The listing builds one solid part. Answer for the finished solid, in the listing's coordinates (mm). Give positions to 0.01 mm unless a question says otherwise; leave off trailing zeros. Loops run counter-clockwise (first coordinate to the right, second up) from the corner with the lowest first, then second, coordinate; pieces in that order, holes last. Notation, with made-up numbers: (14.25, 20) - (54.25, 20) arc R21 ccw to (54.25, 46) - close; hole circle Ø8 at (-25.75, -2.5). An arc over 180 degrees is marked (long way). Write each question's results on one line, items separated by ' | '.
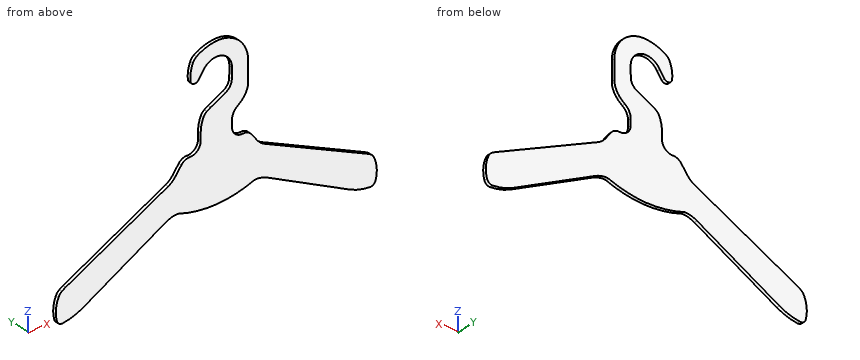
from build123d import *

# Parameters (mm, degrees)
F3_DEPTH = 4
F4_DEPTH = 4


with BuildPart() as f3:
    # F1 (on Front) → F3 (new body)
    with BuildSketch(Plane.XZ):
        with BuildLine():
            Line((-44.725054, 105.2), (-52.498164, 94.835853))
            ThreePointArc((-52.498164, 94.835853), (-56.583657, 90.555592), (-61.560664, 87.355393))
            Line((-61.560664, 87.355393), (-192.6875, 23.557777))
            ThreePointArc((-192.6875, 23.557777), (-195.084903, 22.290786), (-197.392505, 20.866785))
            ThreePointArc((-197.392505, 20.866785), (-200.042611, 18.509777), (-201.934068, 15.50962))
            ThreePointArc((-201.934068, 15.50962), (-205.285397, 2.221076), (-203.882736, -11.411582))
            ThreePointArc((-203.882736, -11.411582), (-201.142788, -15.23423), (-196.597382, -16.442223))
            ThreePointArc((-196.597382, -16.442223), (-183.045193, -13.900552), (-170.274075, -8.702432))
            Line((-170.274075, -8.702432), (-64.872076, 47.128487))
            ThreePointArc((-64.872076, 47.128487), (-58.08245, 49.805832), (-50.868805, 50.915129))
            ThreePointArc((-50.868805, 50.915129), (-49.431216, 50.836816), (-48.034631, 50.487038))
            ThreePointArc((-48.034631, 50.487038), (-24.370411, 44.252825), (0, 42.029373))
            ThreePointArc((0, 42.029373), (24.370411, 44.252825), (48.034631, 50.487038))
            ThreePointArc((48.034631, 50.487038), (49.431216, 50.836816), (50.868805, 50.915129))
            ThreePointArc((50.868805, 50.915129), (58.08245, 49.805832), (64.872076, 47.128487))
            Line((64.872076, 47.128487), (170.274075, -8.702432))
            ThreePointArc((170.274075, -8.702432), (183.045193, -13.900552), (196.597382, -16.442223))
            ThreePointArc((196.597382, -16.442223), (201.142788, -15.23423), (203.882736, -11.411582))
            ThreePointArc((203.882736, -11.411582), (205.285397, 2.221076), (201.934068, 15.50962))
            ThreePointArc((201.934068, 15.50962), (200.042611, 18.509777), (197.392505, 20.866785))
            ThreePointArc((197.392505, 20.866785), (195.084903, 22.290786), (192.6875, 23.557777))
            Line((192.6875, 23.557777), (61.560664, 87.355393))
            ThreePointArc((61.560664, 87.355393), (56.583657, 90.555592), (52.498164, 94.835853))
            Line((52.498164, 94.835853), (44.725054, 105.2))
            ThreePointArc((44.725054, 105.2), (40.491617, 108.733126), (35.125054, 110))
            Line((35.125054, 110), (0, 110))
            Line((0, 110), (-35.125054, 110))
            ThreePointArc((-35.125054, 110), (-40.491617, 108.733126), (-44.725054, 105.2))
        make_face()
    extrude(amount=F3_DEPTH)

    # F2 (on Front) → F4 (join)
    with BuildSketch(Plane.XZ):
        with BuildLine():
            ThreePointArc((33, 110), (23.807612, 113.807612), (20, 123))
            Line((20, 123), (20, 131))
            ThreePointArc((20, 131), (21.982577, 138.891463), (27.459489, 144.908875))
            ThreePointArc((27.459489, 144.908875), (31.203117, 147.749038), (34.561641, 151.035616))
            ThreePointArc((34.561641, 151.035616), (39.21699, 158.62718), (40.840753, 167.383179))
            Line((40.840753, 167.383179), (40.840753, 191.46438))
            ThreePointArc((40.840753, 191.46438), (28.75223, 219.648447), (0, 230.31537))
            ThreePointArc((0, 230.31537), (-10.614416, 228.704114), (-20.691802, 225.001649))
            ThreePointArc((-20.691802, 225.001649), (-23.089205, 223.734658), (-25.396808, 222.310657))
            ThreePointArc((-25.396808, 222.310657), (-28.082385, 219.911622), (-29.982966, 216.85295))
            ThreePointArc((-29.982966, 216.85295), (-32.817521, 207.16869), (-33.099611, 197.082064))
            ThreePointArc((-33.099611, 197.082064), (-29.17364, 192.282166), (-23.222911, 194.026042))
            ThreePointArc((-23.222911, 194.026042), (-20.00524, 198.150829), (-17.110942, 202.508616))
            ThreePointArc((-17.110942, 202.508616), (5.426392, 211.361001), (20.048406, 192.060927))
            Line((20.048406, 192.060927), (19.880676, 178.809665))
            ThreePointArc((19.880676, 178.809665), (17.630944, 171.242723), (11.74383, 165.983274))
            Line((11.74383, 165.983274), (-7.299279, 156.718162))
            ThreePointArc((-7.299279, 156.718162), (-9.696682, 155.45117), (-12.004284, 154.027169))
            ThreePointArc((-12.004284, 154.027169), (-14.654389, 151.670161), (-16.545846, 148.670005))
            ThreePointArc((-16.545846, 148.670005), (-19.126786, 140.786151), (-20, 132.536671))
            Line((-20, 132.536671), (-20, 123))
            ThreePointArc((-20, 123), (-23.807612, 113.807612), (-33, 110))
            Line((-33, 110), (33, 110))
        make_face()
    extrude(amount=F4_DEPTH)


solid = f3.part
Item 1: A cutting plane is placed at C-C, the plane x = -79. Determine the outline of the cut face in (y, z) (3 decimals).
Values found:
outline: (-4, 39.645) - (0, 39.645) - (0, 78.871) - (-4, 78.871) - close
Item 2: A cutting plane is placed at B-B, the plane x = 118. Determine the outline of the cut face in (y, z), plus the area to 3 significant figures.
Values found:
outline: (-4, 18.99) - (0, 18.99) - (0, 59.9) - (-4, 59.9) - close | area: 164 mm²
Item 3: A cutting plane is placed at A-A, the plane z = 31. Determine the outline of the cut face in (x, y), plus the area to 3 significant figures.
Values found:
outline: (-177.39, -4) - (-95.32, -4) - (-95.32, 0) - (-177.39, 0) - close; (95.32, -4) - (177.39, -4) - (177.39, 0) - (95.32, 0) - close | area: 657 mm²
Item 4: Find the intervals of material crossed by line 1 along X through (y, z) = (-3, 14.5); line 2 along X through (y, z) = (-3, 179); line 3 along Z through (x, y) = (31, -0.15), in increasing order. Write a range as [from, to].
Values found:
line 1: x = [-202.37, -126.47], [126.47, 202.37] | line 2: x = [19.88, 40.84] | line 3: z = [45.58, 110.15], [147.58, 217.32]
Item 5: Flat-ended cylindrical pins translate along their axes: P1, Ø1.5, axis at y = -1, z = 28, coming from the -X side; P2, Ø0.6, axis at x = 34, y = -1, coming from the +Z side; P3, Ø1.5, axis at y = -1, z = 46, coming from the -X side; P4, Ø12, axis at x = -46, z = 39, coming from the +Y side. Find the tip coordinate at first contact, or state that the pin passes through.
Values found:
P1: stops at x = -185.1 | P2: stops at z = 213.93 | P3: stops at x = -148.1 | P4: passes through
